Part model, mm, in its own coordinate system. Face numbers are marked on the shaded views. A direction names the side the tool comes from. Give positions to 0.01 mm unless a question says otherwise; leave off trailing zeros. Loops run counter-clockwise (first coordinate to the right, second up) from the corner with the lowest first, then second, coordinate; pieces in that order, holes last. Notation, with made-up numbers: M 6.5,44.25 L 46.5,44.25 A23 ccw 46.5,76.25 Z; hole C 37.5,-14 d1. An arc over 180 degrees is marked long. Answer in a Markdown table with one row per item.
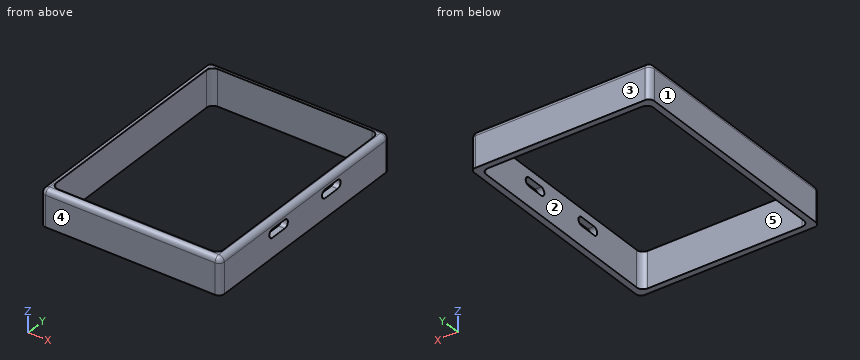
from build123d import *

# Parameters (mm, degrees)
SKETCH010_W     = 84.5
SKETCH010_H     = 109
SKETCH010_W_2   = 78.5
SKETCH010_H_2   = 103
PAD004_DEPTH    = 17
FILLET_R        = 3
FILLET002_R     = 2.5
POCKET025_DEPTH = 9.5


with BuildPart() as part:
    # Sketch010 → Pad004 (new body)
    with BuildSketch(Plane.XY):
        with Locations((4.75, 6.5)):
            Rectangle(SKETCH010_W, SKETCH010_H)
        with Locations((4.75, 6.5)):
            Rectangle(SKETCH010_W_2, SKETCH010_H_2, mode=Mode.SUBTRACT)
    extrude(amount=-PAD004_DEPTH)

    # Fillet
    fillet_edges = [part.edges().sort_by_distance(p)[0] for p in [
        (-34.5, 58, -8.5),
        (-34.5, -45, -8.5),
        (44, 58, -8.5),
        (44, -45, -8.5),
    ]]
    fillet(fillet_edges, radius=FILLET_R)

    # Fillet002
    fillet002_edges = [part.edges().sort_by_distance(p)[0] for p in [
        (47, 61, -8.5),
        (-37.5, 61, -8.5),
        (47, -48, -8.5),
        (-37.5, -48, -8.5),
        (-37.5, 6.5, 0),
        (4.75, -48, 0),
        (47, 6.5, 0),
        (4.75, 61, 0),
    ]]
    fillet(fillet002_edges, radius=FILLET002_R)

    # Sketch058 → Pocket025 (cut, symmetric)
    with BuildSketch(Plane.YZ.offset(41)):
        with BuildLine():
            ThreePointArc((-14.532044, -3.85902), (-16.532044, -5.85902), (-14.532044, -7.85902))
            Line((-14.532044, -7.85902), (-6.532044, -7.85902))
            ThreePointArc((-6.532044, -7.85902), (-4.532044, -5.85902), (-6.532044, -3.85902))
            Line((-6.532044, -3.85902), (-14.532044, -3.85902))
        make_face()
        with BuildLine():
            ThreePointArc((19.467956, -3.85902), (17.467956, -5.85902), (19.467956, -7.85902))
            Line((19.467956, -7.85902), (27.467956, -7.85902))
            ThreePointArc((27.467956, -7.85902), (29.467956, -5.85902), (27.467956, -3.85902))
            Line((27.467956, -3.85902), (19.467956, -3.85902))
        make_face()
    extrude(amount=POCKET025_DEPTH, both=True, mode=Mode.SUBTRACT)


with BuildPart() as part_1:
    # Body005 placement: moved
    add(part.part.moved(Location((0, 0, 4.5))))


solid = part_1.part
(1) Drill centre lines: line 1 along Y through (x, z) = (-28, -8.25); line 2 along X through (y, z) = (35, -10.5); line 3 along X through (y, z) = (49.5, 3). Where is each one in solid material? Low to high.
Recorded:
| item | result |
|---|---|
| line 1 | y = -48 to -45, 58 to 61 |
| line 2 | x = -37.5 to -34.5, 44 to 47 |
| line 3 | x = -37.29 to -34.5, 44 to 46.79 |
(2) Which spindle directions (+Z, -Z, +X, -X, +Y, -Y) get a long thin tool onto all of the face, cutting with end or side? Do the marked faces 4 and 5. Say none if no direction does.
Recorded:
| item | result |
|---|---|
| face 4 | +Z, -Z, +X, -X, -Y |
| face 5 | +Z, -Z |
(3) Saw through at A-A (x = 24). Write the cut outline in (y, z).
Recorded:
| item | result |
|---|---|
| outline | M -48,-12.5 L -45,-12.5 L -45,4.5 L -45.5,4.5 A2.5 ccw -48,2 Z; M 58,-12.5 L 61,-12.5 L 61,2 A2.5 ccw 58.5,4.5 L 58,4.5 Z |
(4) Pull direction Y, two halves, no side cores. Call the marked faces 1, 2 and 3: +Y half, -Y half, draft (parallel to the pull), parting line (faces both ways), or undercut.
Recorded:
| item | result |
|---|---|
| face 1 | draft |
| face 2 | undercut |
| face 3 | +Y half |
(5) Saw through at B-B (z = -5). Write the cut outline in (x, y).
Recorded:
| item | result |
|---|---|
| outline | M -37.5,-45.5 A2.5 ccw -35,-48 L 44.5,-48 A2.5 ccw 47,-45.5 L 47,58.5 A2.5 ccw 44.5,61 L -35,61 A2.5 ccw -37.5,58.5 Z; hole M -34.5,-42 A3 ccw -31.5,-45 L 41,-45 A3 ccw 44,-42 L 44,55 A3 ccw 41,58 L -31.5,58 A3 ccw -34.5,55 Z |
(6) Saw through at C-C (y = -34). Write the cut outline in (x, z).
Recorded:
| item | result |
|---|---|
| outline | M -37.5,-12.5 L -34.5,-12.5 L -34.5,4.5 L -35,4.5 A2.5 ccw -37.5,2 Z; M 44,-12.5 L 47,-12.5 L 47,2 A2.5 ccw 44.5,4.5 L 44,4.5 Z |
(7) Saw through at D-D (z = 3.25). Write the cut outline in (x, y).
Recorded:
| item | result |
|---|---|
| outline | M -37.17,-45.5 A2.17 ccw -35,-47.67 L 44.5,-47.67 A2.17 ccw 46.67,-45.5 L 46.67,58.5 A2.17 ccw 44.5,60.67 L -35,60.67 A2.17 ccw -37.17,58.5 Z; hole M -34.5,-42 A3 ccw -31.5,-45 L 41,-45 A3 ccw 44,-42 L 44,55 A3 ccw 41,58 L -31.5,58 A3 ccw -34.5,55 Z |
